Check sheet for the modelled part. Datum: model origin and axes. Units: mm. A direction names the side the tool comes from. Round coordinates to 2 decimals unless told otherwise and drop trailing zeros. Order: outer loops, then holes, each group sorted by start corner. A loop starts at its lowest first (then second) coordinate and runs counter-clockwise, first axis right, second up.
(1) Depth check by flat-ended pin: pin 1 (5 mm diameter, centred on y = 13, z = 9, fed in from +X); pin 2 (1 mm diameter, centred on x = -9.5, z = 9.5, fed in from +Y); pin 3 (1.6 mm diameter, centred on x = -9, z = 9.5, fed in from -Y). Enter the tip coordinate at first touch or a pass-through.
(2) Tool access check on faces 1 (the flat face through (-26.447, 13, 16)), 2 (the flat face through (-8.039, 13, 5)), 3 (the flat face through (-23, 13, 5.169)), 4 (the flat face through (-24, 27.692, 4)), 5 (the flat face through (-10.097, 33, 10)). Record the directions out of +Z, -Z, +X, -X, +Y, -Y that give a thin tool (end or side, any length) a straight path to the whole face; none if there is none.
(3) Thickness scan on probe 1 along X at (y, z) = (21, 19); probe 2 along Y at (x, z) = (5.5, 3.25); probe 3 along Z at (x, y) = (-10, -8). Record the ranges inside material, lowest first.
(4) Mould release check, pull along Z, two halves, no side actions. Record for faces 6 (the flat face through (-15, 7, 19.863)), 7 (the flat face through (-24, -2.28, 4)), 8 (the flat face through (-21.844, 3.437, 13.137)), 9 (the flat face through (1, -8, 12.243)): released by +Z, released by -Z, zero draft, split by the parting line, or undercut.
(5) Sectioned sample at C-C, the plane y = 24. Enter the section's corners in (x, z).
(6) Sectioned sample at B-B, the plane z = 18. Enter the section's corners in (x, y).
(7) Sectioned sample at A-A, the plane x = 2. Enter the section's corners in (y, z).
```python
from build123d import *

# Parameters (mm, degrees)
SERVO_CLASPER_2ND_HALF_SERVO_A_DEPTH     = 7.62
CUTOUT_START                             = 7.62
CENTER_ENCAPSULATOR_W                    = 2.0574
CENTER_ENCAPSULATOR_H                    = 12.446
CENTER_ENCAPSULATOR_H_2                  = 12.377096657
CUTOUT_TO_HOLD_SERVO_DEPTH               = 4.6228
SERVO_START                              = 12.2428
SERVO_CLASPER_2ND_HALF_OTHER_SERVO_DEPTH = 7.62
SKETCH12_W                               = 19.8628
SKETCH12_H                               = 45.212
SERVO_HOLDER_EXTRUDE_DEPTH               = 16.350000066
SERVO_B_CUT_DEPTH                        = 7.62
SERVO_B_SECURER_CUT_DEPTH                = 49.383140951
SERVO_B_SECURER_CUT_DEPTH_BACK           = 49.383140951
SKETCH18_W                               = 2.032
SKETCH18_H                               = 8.21582812


with BuildPart() as part:
    # Sketch1 → Servo Clasper 2nd Half (Servo A) (new body)
    with BuildSketch(Plane.XY):
        Polygon((12.25510559, 35.312310559), (12.25510559, 32.772310559), (-8.03949441, 32.772310559), (-8.03949441, -7.359689441), (12.25510559, -7.359689441), (12.25510559, -9.899689441), (-10.09689441, -9.899689441), (-10.09689441, 35.312310559), align=None)
    extrude(amount=SERVO_CLASPER_2ND_HALF_SERVO_A_DEPTH)

    # center encapsulator → Cutout to hold servo (add)
    with BuildSketch(Plane.XY.offset(CUTOUT_START)):
        with Locations((-9.06819441, 24.072810559)):
            Rectangle(CENTER_ENCAPSULATOR_W, CENTER_ENCAPSULATOR_H)
        with Locations((-9.06819441, 1.374262231)):
            Rectangle(CENTER_ENCAPSULATOR_W, CENTER_ENCAPSULATOR_H_2)
    extrude(amount=CUTOUT_TO_HOLD_SERVO_DEPTH)

    # Sketch7 → Servo Clasper 2nd Half (Other Servo) (add)
    with BuildSketch(Plane.XY.offset(SERVO_START)):
        Polygon((12.25510559, 35.312310559), (12.25510559, 32.772310559), (-8.03949441, 32.772310559), (-8.03949441, -7.359689441), (12.25510559, -7.359689441), (12.25510559, -9.899689441), (-10.09689441, -9.899689441), (-10.09689441, 35.312310559), align=None)
    extrude(amount=SERVO_CLASPER_2ND_HALF_OTHER_SERVO_DEPTH)

    # Sketch12 → Servo Holder Extrude (add)
    with BuildSketch(Plane.ZY.offset(10.09689441)):
        with Locations((9.9314, 12.706310559)):
            Rectangle(SKETCH12_W, SKETCH12_H)
    extrude(amount=SERVO_HOLDER_EXTRUDE_DEPTH)

    # Sketch14 → Servo B Cut (cut)
    with BuildSketch(Plane.ZY.offset(26.446894476)):
        Polygon((7.29615, 29.470310559), (12.05865, 29.470310559), (14.1859, 14.687510559), (14.1859, 10.725110559), (12.05865, -4.057689441), (7.29615, -4.057689441), (5.1689, 10.725110559), (5.1689, 14.687510559), align=None)
    extrude(amount=-SERVO_B_CUT_DEPTH, mode=Mode.SUBTRACT)

    # Sketch18 → Servo B Securer Cut (cut, two sides: drawn at the far end of the back side and taken through both)
    with BuildSketch(Plane(origin=(0, 0, 0), x_dir=(-1, 0, 0), z_dir=(0, 0, -1)).offset(-SERVO_B_SECURER_CUT_DEPTH_BACK)):
        with Locations((23.652894476, 23.584396499)):
            Rectangle(SKETCH18_W, SKETCH18_H)
        Polygon((24.668894476, 5.874578093), (22.636894476, 5.936138467), (22.636894476, -2.279689441), (24.668894476, -2.279689441), align=None)
    extrude(amount=SERVO_B_SECURER_CUT_DEPTH + SERVO_B_SECURER_CUT_DEPTH_BACK, mode=Mode.SUBTRACT)


solid = part.part
```
Derived:
1. pin 1: stops at x = -8.04
1. pin 2: stops at y = 30.3
1. pin 3: stops at y = -4.81
2. face 1: +Z, -Z, -X, +Y, -Y
2. face 2: +Z, -Z, +X
2. face 3: -X
2. face 4: +Z, -Z
2. face 5: +X, +Y
3. probe 1: x = -26.45 to -24.67, -22.64 to -8.04
3. probe 2: y = -9.9 to -7.36, 32.77 to 35.31
3. probe 3: z = 0 to 7.62, 12.24 to 19.86
4. face 6: released by +Z
4. face 7: zero draft
4. face 8: undercut
4. face 9: undercut
5. outline: (-26.45, 0) - (-24.67, 0) - (-24.67, 6.51) - (-26.45, 6.51) - close; (-26.45, 12.85) - (-24.67, 12.85) - (-24.67, 19.86) - (-26.45, 19.86) - close; (-22.64, 0) - (-8.04, 0) - (-8.04, 19.86) - (-22.64, 19.86) - (-22.64, 12.85) - (-18.83, 12.85) - (-18.83, 6.51) - (-22.64, 6.51) - close
6. outline: (-26.45, -9.9) - (12.26, -9.9) - (12.26, -7.36) - (-8.04, -7.36) - (-8.04, 32.77) - (12.26, 32.77) - (12.26, 35.31) - (-26.45, 35.31) - close; hole (-24.67, -2.28) - (-22.64, -2.28) - (-22.64, 5.94) - (-24.67, 5.87) - close; hole (-24.67, 19.48) - (-22.64, 19.48) - (-22.64, 27.69) - (-24.67, 27.69) - close
7. outline: (-9.9, 0) - (-7.36, 0) - (-7.36, 7.62) - (-9.9, 7.62) - close; (-9.9, 12.24) - (-7.36, 12.24) - (-7.36, 19.86) - (-9.9, 19.86) - close; (32.77, 0) - (35.31, 0) - (35.31, 7.62) - (32.77, 7.62) - close; (32.77, 12.24) - (35.31, 12.24) - (35.31, 19.86) - (32.77, 19.86) - close
